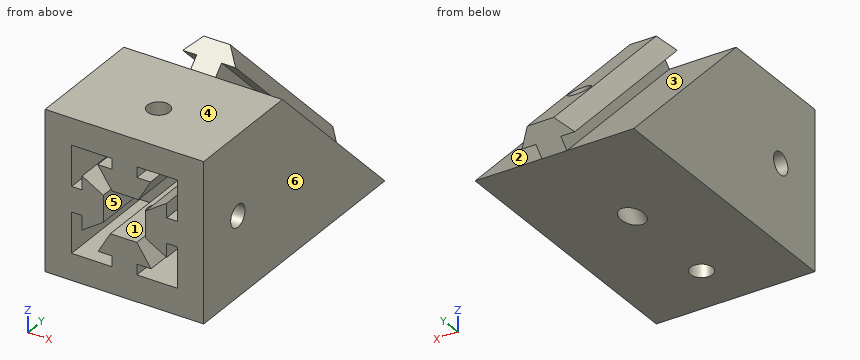
```python
from build123d import *

# Parameters (mm, degrees)
SKETCH1_W           = 30
SKETCH1_H           = 30
SKETCH1_W_2         = 20
SKETCH1_H_2         = 20
BOSS_EXTRUDE1_DEPTH = 20
SKETCH2_W           = 4.711017494
SKETCH2_H           = 2
SKETCH2_W_2         = 2
SKETCH2_H_2         = 4.711017494
BOSS_EXTRUDE2_DEPTH = 20
SKETCH3_R           = 2.1
CUT_EXTRUDE1_DEPTH  = 31
SKETCH4_R           = 2.1
CUT_EXTRUDE2_DEPTH  = 31
BOSS_EXTRUDE3_DEPTH = 30
SKETCH8_W           = 4.711017494
SKETCH8_H           = 2.5
BOSS_EXTRUDE4_DEPTH = 42.42640687
SKETCH9_R           = 2.1
CUT_EXTRUDE3_DEPTH  = 44.261940705


with BuildPart() as part:
    # Sketch1 → Boss-Extrude1 (new body)
    with BuildSketch(Plane(origin=(0, 0, 0), x_dir=(1, 0, 0), z_dir=(0, 1, 0))):
        Rectangle(SKETCH1_W, SKETCH1_H)
        Rectangle(SKETCH1_W_2, SKETCH1_H_2, mode=Mode.SUBTRACT)
    extrude(amount=BOSS_EXTRUDE1_DEPTH)


with BuildPart() as body_2:
    # Sketch2 → Boss-Extrude2 (new body)
    with BuildSketch(Plane(origin=(0, 20, 0), x_dir=(1, 0, 0), z_dir=(0, 1, 0))):
        Polygon((2.336539675, 4), (-2.663460325, 4), (-4.950152781, 8), (5.049847219, 8), align=None)
        with Locations((0, 9)):
            Rectangle(SKETCH2_W, SKETCH2_H)
        Polygon((-4, 2.336539675), (-4, -2.663460325), (-8, -4.950152781), (-8, 5.049847219), align=None)
        Polygon((-2.336539675, -4), (2.663460325, -4), (4.950152781, -8), (-5.049847219, -8), align=None)
        with Locations((0, -9)):
            Rectangle(SKETCH2_W, SKETCH2_H)
        Polygon((4, 2.663460325), (4, -2.336539675), (8, -5.049847219), (8, -2.355508747), (8, 2.355508747), (8, 4.950152781), align=None)
        with Locations((9, 0)):
            Rectangle(SKETCH2_W_2, SKETCH2_H_2)
        with Locations((-9, 0)):
            Rectangle(SKETCH2_W_2, SKETCH2_H_2)
    extrude(amount=-BOSS_EXTRUDE2_DEPTH)


with BuildPart() as cut_extrude1_tool:
    # Sketch3 → Cut-Extrude1 (new body, through all)
    with BuildSketch(Plane.ZY.offset(15)):
        with Locations((0, 10)):
            Circle(SKETCH3_R)
    extrude(amount=-CUT_EXTRUDE1_DEPTH)


with BuildPart() as part_1:
    add(part.part)

    # Cut-Extrude1: cut by cut_extrude1_tool
    add(cut_extrude1_tool.part, mode=Mode.SUBTRACT)


with BuildPart() as body_2_1:
    add(body_2.part)

    # Cut-Extrude1: cut by cut_extrude1_tool
    add(cut_extrude1_tool.part, mode=Mode.SUBTRACT)


with BuildPart() as cut_extrude2_tool:
    # Sketch4 → Cut-Extrude2 (new body, through all)
    with BuildSketch(Plane(origin=(0, 0, -15), x_dir=(-1, 0, 0), z_dir=(0, 0, -1))):
        with Locations((0, 10)):
            Circle(SKETCH4_R)
    extrude(amount=-CUT_EXTRUDE2_DEPTH)


with BuildPart() as part_2:
    add(part_1.part)

    # Cut-Extrude2: cut by cut_extrude2_tool
    add(cut_extrude2_tool.part, mode=Mode.SUBTRACT)



with BuildPart() as body_2_2:
    add(body_2_1.part)

    # Cut-Extrude2: cut by cut_extrude2_tool
    add(cut_extrude2_tool.part, mode=Mode.SUBTRACT)


with BuildPart() as part_3:
    add(part_2.part)

    add(body_2_2.part)  # Boss-Extrude3 merges body 2
    # Sketch5 → Boss-Extrude3 (add)
    with BuildSketch(Plane(origin=(15, 0, 0), x_dir=(0, 0, -1), z_dir=(1, 0, 0))):
        Polygon((15, 53.049895295), (15, 50), (-15, 20), (-15, 23.049895295), align=None)
        Polygon((15, 50), (-15, 20), (15, 20), align=None)
    extrude(amount=-BOSS_EXTRUDE3_DEPTH)

    # Sketch8 → Boss-Extrude4 (add)
    with BuildSketch(Plane(origin=(0, 34.024947648, -34.024947648), x_dir=(1, 0, 0), z_dir=(0, -0.707106781, 0.707106781))):
        Polygon((2.5, 32.655338987), (-2.5, 32.655338987), (-4.999999998, 29.405338987), (-2.355508747, 29.405338987), (2.355508747, 29.405338987), (5.000000002, 29.405338987), align=None)
        with Locations((0, 28.155338987)):
            Rectangle(SKETCH8_W, SKETCH8_H)
    extrude(amount=BOSS_EXTRUDE4_DEPTH)

    # Sketch9 → Cut-Extrude3 (cut, through all)
    with BuildSketch(Plane(origin=(0, 23.090811639, 23.090811639), x_dir=(1, 0, 0), z_dir=(0, 0.707106781, 0.707106781))):
        with Locations((0, 31.96811151)):
            Circle(SKETCH9_R)
    extrude(amount=-CUT_EXTRUDE3_DEPTH, mode=Mode.SUBTRACT)


solid = part_3.part
```
For this review, take the finished solid that the model builds, in its own axes (mm). Face numbers are marked on the shaded views. A direction names the side the tool comes from. Round coordinates to 2 decimals unless told otherwise and drop trailing zeros. Write each loop counter-clockwise with the first axis right and the second up, starting at its lowest first coordinate (ties: lowest second). Pieces come first, ordered by that corner, then holes. Notation, with made-up numbers: (19.5, 29) - (27.5, 29) arc R17 cw to (27.5, 42) - close; hole circle Ø1 at (-40, 89.25). An arc over 180 degrees is marked (long way). Use CSV: the item, a comma, the result in double quotes.
1) For the marked faces 1, 2 and 3, list the 3-axis set-ups (+Z, -Z, +X, -X, +Y, -Y) from which the entire face can be reached by the end or side of a thin tool; tool diameter is ignored.
Conclusion:
face 1,"-Y"
face 2,"+X"
face 3,"-X"
2) The part is to be moulded in two halves that separate along Z. For the marked faces 4, 5 and 6, say which applies: pulls with the +Z half, pulls with the -Z half, needs draft (parallel to the pull), parting line crosses it, or undercut.
Conclusion:
face 4,"pulls with the +Z half"
face 5,"undercut"
face 6,"needs draft"
3) Add section C-C on x = 0. Write out the cut boundary in (y, z), and give its area (3 significant figures).
Conclusion:
outline,"(0, -15) - (7.9, -15) - (7.9, -4) - (0, -4) - close; (0, 4) - (7.9, 4) - (7.9, 15) - (0, 15) - close; (12.1, -15) - (27.24, -15) - (44.21, 1.97) - (27.12, 19.07) - (23.05, 15) - (12.1, 15) - (12.1, 4) - (20, 4) - (20, -4) - (12.1, -4) - close; (33.18, -15) - (53.05, -15) - (57.12, -10.93) - (47.18, -1) - close"
area,"1,040 mm^2"
4) Wall thickness on line 1 along Z through (x, y) = (1, 2.5); line 2 along Z through (x, y) = (-6.5, 3.5); line 3 along Y through (x, z) = (0, -6.75): over which ranges is each line inside the solid? List them lowest first. Write a range as from..to.
Conclusion:
line 1,"z = -15..-4, 4..15"
line 2,"z = -15..-10, -4.03..4.09, 10..15"
line 3,"y = 0..7.9, 12.1..35.49, 41.43..52.93"
5) Clearance check with flat-ended pins moving along their axes: pin 1 Ø2 at (y, z) = (44.5, -3.5) entering from +X; pin 2 Ø6 at (x, y) = (-6, 17.5) entering from +Z; pin 3 Ø1.5 at (x, y) = (-11.5, 26.5) entering from +Z. State where each tip first meets the part, or that it passes through.
Conclusion:
pin 1,"stops at x = 5"
pin 2,"stops at z = 15"
pin 3,"stops at z = 12.3"
6) Add section B-B on z = 13.5. Write out the cut boundary in (x, y), and give its area (3 significant figures).
Conclusion:
outline,"(-15, 0) - (15, 0) - (15, 24.55) - (2.36, 24.55) - (2.36, 28.09) - (5, 28.09) - (2.5, 32.68) - (-2.5, 32.68) - (-5, 28.09) - (-2.36, 28.09) - (-2.36, 24.55) - (-15, 24.55) - close; hole circle Ø4.2 at (0, 10)"
area,"774 mm^2"
7) Add section A-A on x = -9. Write out the cut boundary in (y, z), and give its area (3 significant figures).
Conclusion:
outline,"(0, -15) - (53.05, -15) - (23.05, 15) - (0, 15) - (0, 10) - (20, 10) - (20, 2.36) - (0, 2.36) - (0, -2.36) - (20, -2.36) - (20, -10) - (0, -10) - close; hole circle Ø4.2 at (10, 0)"
area,"822 mm^2"
8) Add section D-D on y = 10. Count the separate pieces of the cut face and the enclosed holes in it, and give its area (3 significant figures).
Conclusion:
separate pieces,"4"
enclosed holes,"0"
area,"473 mm^2"
